```python
from build123d import *

# Parameters (mm, degrees)
SKETCH1_W           = 200
SKETCH1_H           = 200
BOSS_EXTRUDE1_DEPTH = 10
SHELL1_T            = -2.5
SKETCH2_W           = 100
SKETCH2_H           = 100
CUT_EXTRUDE1_DEPTH  = 142.620090383


with BuildPart() as part:
    # Sketch1 → Boss-Extrude1 (new body)
    with BuildSketch(Plane(origin=(0, 0, 0), x_dir=(1, 0, 0), z_dir=(0, 1, 0))):
        Rectangle(SKETCH1_W, SKETCH1_H)
    extrude(amount=BOSS_EXTRUDE1_DEPTH)

    # Shell1
    shell1_openings = [part.faces().sort_by_distance(p)[0] for p in [
        (0, 10, 0),
    ]]
    offset(amount=SHELL1_T, openings=shell1_openings, kind=Kind.INTERSECTION)

    # Sketch2 → Cut-Extrude1 (cut, through all)
    with BuildSketch(Plane(origin=(0, 2.5, 0), x_dir=(1, 0, 0), z_dir=(0, 1, 0))):
        Rectangle(SKETCH2_W, SKETCH2_H)
    extrude(amount=-CUT_EXTRUDE1_DEPTH, mode=Mode.SUBTRACT)


solid = part.part
```
Can you work these out from the model? Positions are in its coordinate system, mm. A direction names the side the tool comes from. Coordinates: 2 decimals unless noted, no trailing zeros. Loops run counter-clockwise (first coordinate to the right, second up) from the corner with the lowest first, then second, coordinate; pieces in that order, holes last. Notation, with made-up numbers: (20.5, 63) - (47.5, 63) arc R32 ccw to (47.5, 100) - close; hole circle Ø4 at (9, 52). An arc over 180 degrees is marked (long way). Use a Markdown table: item, result.
Item 1: I want a section at A-A on z = 37. Please give me the cut outline in (x, y), and give its area (4 significant figures).
Numbers:
| item | result |
|---|---|
| outline | (-100, 0) - (-50, 0) - (-50, 2.5) - (-97.5, 2.5) - (-97.5, 10) - (-100, 10) - close; (50, 0) - (100, 0) - (100, 10) - (97.5, 10) - (97.5, 2.5) - (50, 2.5) - close |
| area | 287.5 mm2 |
Item 2: I want a section at B-B on y = 4. Please give me the cut outline in (x, z), and give its area (4 significant figures).
Numbers:
| item | result |
|---|---|
| outline | (-100, -100) - (100, -100) - (100, 100) - (-100, 100) - close; hole (-97.5, -97.5) - (97.5, -97.5) - (97.5, 97.5) - (-97.5, 97.5) - close |
| area | 1,975 mm2 |
Item 3: If I drill on probe 1 along Z at (x, y) = (67, 8); probe 2 along X at (y, z) = (0.5, 30.5), over which ranges is the centre line in solid material (lowest first)? Write a range as from..to.
Numbers:
| item | result |
|---|---|
| probe 1 | z = -100..-97.5, 97.5..100 |
| probe 2 | x = -100..-50, 50..100 |
Item 4: I want a section at C-C on x = 42. Please give me the cut outline in (y, z).
Numbers:
| item | result |
|---|---|
| outline | (0, -100) - (10, -100) - (10, -97.5) - (2.5, -97.5) - (2.5, -50) - (0, -50) - close; (0, 50) - (2.5, 50) - (2.5, 97.5) - (10, 97.5) - (10, 100) - (0, 100) - close |
Item 5: Will this pin go through, and if not, where does the flat tip stop? pin 1 (6 mm diameter, centred on x = 58.5, z = 34.5, fed in from +Y).
Numbers:
| item | result |
|---|---|
| pin 1 | stops at y = 2.5 |
Item 6: For faces 1 (the face through (-97.5, 6, 1)), 2 (the face through (-100, 5, 1)), which set-ups out of +Z, -Z, +X, -X, +Y, -Y let a thin tool reach every point of the face, with its end or its side?
Numbers:
| item | result |
|---|---|
| face 1 | +Y |
| face 2 | +Z, -Z, -X, +Y, -Y |
Item 7: We'd pull the mould along Z, two halves only. Please class faces 3 (the face through (100, 5, 1)), 4 (the face through (-1, 5, 100)), 5 (the face through (-66, 2.5, -1)): released by +Z, released by -Z, zero draft, split by the parting line, or undercut.
Numbers:
| item | result |
|---|---|
| face 3 | zero draft |
| face 4 | released by +Z |
| face 5 | undercut |
Item 8: I want a section at D-D on z = 84.5. Please give me the cut outline in (x, y), and give its area (4 significant figures).
Numbers:
| item | result |
|---|---|
| outline | (-100, 0) - (100, 0) - (100, 10) - (97.5, 10) - (97.5, 2.5) - (-97.5, 2.5) - (-97.5, 10) - (-100, 10) - close |
| area | 537.5 mm2 |
